from build123d import *

# Parameters (mm, degrees)
F0_W       = 225.552
F0_H       = 9.652
F1_DEPTH   = 19.05
F3_D       = 19.05
F5_W       = 6.35
F5_H       = 260.096
F6_DEPTH   = 19.05
F9_D       = 16.002
F10_W      = 50.8
F10_H      = 25.4
F11_DEPTH  = 22.352
F12_SIZE   = 6.35
F14_D      = 7.9375
F16_D      = 10.3124
F16_DEPTH  = 28.8925
F16_TIP    = 3.0981575238
F18_D      = 10.3124
F18_DEPTH  = 12.7
F18_TIP    = 3.0981575238
F20_DEPTH  = 6.35
F22_SIZE   = 14.224
F22_2_SIZE = 14.224
F23_W      = 38.1
F23_H      = 276.225
F24_DEPTH  = 7.874


with BuildPart() as f1:
    # F0 (on Right) → F1 (new body, symmetric)
    with BuildSketch(Plane.YZ):
        with Locations((0, 134.874)):
            Rectangle(F0_W, F0_H)
    extrude(amount=F1_DEPTH, both=True)

    # F3 (through all)
    with Locations(Plane.XY.offset(139.7)):
        with Locations((0, -96.8375), (0, 96.8375)):
            Hole(F3_D / 2)


with BuildPart() as f4_1:
    # F4: instance of F1
    add(f1.part.mirror(Plane.XY))


with BuildPart() as f6:
    # F5 (on Right) → F6 (new body, symmetric)
    with BuildSketch(Plane.YZ):
        with Locations((-80.9625, 0)):
            Rectangle(F5_W, F5_H)
    extrude(amount=F6_DEPTH, both=True)


with BuildPart() as f6b:
    # F5 (on Right) → F6, piece 2 (new body, symmetric)
    with BuildSketch(Plane.YZ):
        with Locations((80.9625, 0)):
            Rectangle(F5_W, F5_H)
    extrude(amount=F6_DEPTH, both=True)


with BuildPart() as f1_1:
    add(f1.part)

    # F8: union F6, F6b, F4_1
    add(f6.part)
    add(f6b.part)
    add(f4_1.part)

    # F9 (through all)
    with Locations(Plane(origin=(0, 84.1375, 0), x_dir=(-1, 0, 0), z_dir=(0, 1, 0))):
        with Locations((0, -3.048)):
            Hole(F9_D / 2)

    # F10 (on face) → F11 (join)
    with BuildSketch(Plane.XY.offset(-130.048)):
        with Locations((0, -51.689)):
            Rectangle(F10_W, F10_H)
        Rectangle(F10_W, F10_H)
        with Locations((0, 51.689)):
            Rectangle(F10_W, F10_H)
    extrude(amount=F11_DEPTH)

    # F12
    f12_edges = [f1_1.edges().sort_by_distance(p)[0] for p in [
        (-25.4, -51.689, -107.696),
        (-25.4, 0, -107.696),
        (-25.4, 51.689, -107.696),
        (25.4, 51.689, -107.696),
        (25.4, 0, -107.696),
        (25.4, -51.689, -107.696),
    ]]
    chamfer(f12_edges, length=F12_SIZE)

    # F14 (through all)
    with Locations(Plane.XY.offset(139.7)):
        with Locations((0, -34.925), (0, 34.925)):
            Hole(F14_D / 2)

    # F16
    with Locations(Plane.XY.offset(139.7)):
        with Locations((0, 0)):
            Hole(F16_D / 2, depth=F16_DEPTH)
            with Locations((0, 0, -(F16_DEPTH + F16_TIP / 2))):  # 118° drill point
                Cone(0, F16_D / 2, F16_TIP, mode=Mode.SUBTRACT)

    # F18
    with Locations(Plane(origin=(0, 0, -139.7), x_dir=(1, 0, 0), z_dir=(0, 0, -1))):
        with Locations((0, 0)):
            Hole(F18_D / 2, depth=F18_DEPTH)
            with Locations((0, 0, -(F18_DEPTH + F18_TIP / 2))):  # 118° drill point
                Cone(0, F18_D / 2, F18_TIP, mode=Mode.SUBTRACT)

    # F21: F20 across plane


with BuildPart() as f20:
    # F19 (on face) → F20 (new body)
    with BuildSketch(Plane.XY.offset(139.7)):
        Polygon((19.05, 104.902), (19.05, 79.502), (73.2887461782, 79.502), (95.25, 79.502), (95.25, 104.902), align=None)
    extrude(amount=-F20_DEPTH)


with BuildPart() as f1_2:
    add(f1_1.part)
    add(f20.part.mirror(Plane.XY))

    # F22#2
    f22_2_edges = [f1_2.edges().sort_by_distance(p)[0] for p in [
        (95.25, 79.502, -136.525),
    ]]
    chamfer(f22_2_edges, length=F22_2_SIZE)



with BuildPart() as f20_1:
    add(f20.part)

    # F22
    f22_edges = [f20_1.edges().sort_by_distance(p)[0] for p in [
        (95.25, 79.502, 136.525),
    ]]
    chamfer(f22_edges, length=F22_SIZE)


with BuildPart() as f1_3:
    add(f1_2.part)

    add(f20_1.part)  # F24 merges F20
    # F23 (on face) → F24 (join)
    with BuildSketch(Plane(origin=(0, 104.902, 0), x_dir=(-1, 0, 0), z_dir=(0, 1, 0))):
        with Locations((-76.2, -1.5875)):
            Rectangle(F23_W, F23_H)
    extrude(amount=F24_DEPTH)


solid = f1_3.part
Read the model definition and answer for the solid it produces. Units are mm, in the model's axes. A direction names the side the tool comes from. Round coordinates to 2 decimals unless told otherwise and drop trailing zeros. Write each loop counter-clockwise with the first axis right and the second up, starting at its lowest first coordinate (ties: lowest second). Pieces come first, ordered by that corner, then holes. Notation, with made-up numbers: M 4,-15.5 L 56,-15.5 A15 cw 56,6.5 Z; hole C -15,-26.75 d4. An arc over 180 degrees is marked long. Use a Markdown table: item, result.
1) The part is cut by section B-B (z = -97.5). Write down the section's boundary in (x, y), plus the area to 3 significant figures.
Answers follow:
| item | result |
|---|---|
| outline | M -19.05,-84.14 L 19.05,-84.14 L 19.05,-77.79 L -19.05,-77.79 Z; M -19.05,77.79 L 19.05,77.79 L 19.05,84.14 L -19.05,84.14 Z; M 57.15,104.9 L 95.25,104.9 L 95.25,112.78 L 57.15,112.78 Z |
| area | 784 mm2 |
2) The part is cut by section D-D (x = 34). Write down the section's boundary in (y, z).
Answers follow:
| item | result |
|---|---|
| outline | M 79.5,-139.7 L 104.9,-139.7 L 104.9,-133.35 L 79.5,-133.35 Z; M 79.5,133.35 L 104.9,133.35 L 104.9,139.7 L 79.5,139.7 Z |
3) The part is cut by section A-A (y = 42.5). Write down the section's boundary in (x, z), plus the area to 3 significant figures.
Answers follow:
| item | result |
|---|---|
| outline | M -25.4,-130.05 L -19.05,-130.05 L -19.05,-139.7 L 19.05,-139.7 L 19.05,-130.05 L 25.4,-130.05 L 25.4,-114.05 L 19.05,-107.7 L -19.05,-107.7 L -25.4,-114.05 Z; M -19.05,130.05 L 19.05,130.05 L 19.05,139.7 L -19.05,139.7 Z |
| area | 1,830 mm2 |
4) For a pull along Y with two mould halves and no side action, classify faces 5 (the flat face through (0, -112.776, 135)), 6 (the flat face through (0, 26, -130.048)), 7 (the flat face through (0, 112.776, 135)), 8 (the flat face through (9, 101, 130.048)) as pulls with the +Y half, pulls with the -Y half, needs draft (parallel to the pull), parting line crosses it, or undercut.
Answers follow:
| item | result |
|---|---|
| face 5 | pulls with the -Y half |
| face 6 | undercut |
| face 7 | pulls with the +Y half |
| face 8 | needs draft |
5) A tool of negligible diameter and unlimited length cuts with its end or side. For faces 1 (the flat face through (50, 79.502, -137)), 2 (the flat face through (0, 52, -107.696)), 3 (the flat face through (76, 109, 136.525)), 4 (the flat face through (9, -102, 130.048)), from which of +Z, -Z, +X, -X, +Y, -Y can it reach the whole face along a straight path? Write none if from no direction.
Answers follow:
| item | result |
|---|---|
| face 1 | +Z, -Z, +X, -Y |
| face 2 | +X, -X |
| face 3 | +Z, +X, +Y |
| face 4 | +X, -X, -Y |
6) The part is cut by section C-C (x = 14). Write down the section's boundary in (y, z), plus the area to 3 significant figures.
Answers follow:
| item | result |
|---|---|
| outline | M -112.78,-139.7 L 112.78,-139.7 L 112.78,-130.05 L 84.14,-130.05 L 84.14,130.05 L 112.78,130.05 L 112.78,139.7 L -112.78,139.7 L -112.78,130.05 L -84.14,130.05 L -84.14,-130.05 L -112.78,-130.05 Z; hole M -77.79,-130.05 L -64.39,-130.05 L -64.39,-107.7 L -38.99,-107.7 L -38.99,-130.05 L -12.7,-130.05 L -12.7,-107.7 L 12.7,-107.7 L 12.7,-130.05 L 38.99,-130.05 L 38.99,-107.7 L 64.39,-107.7 L 64.39,-130.05 L 77.79,-130.05 L 77.79,130.05 L -77.79,130.05 Z |
| area | 9,360 mm2 |
7) Flat-ended cylindrical pins translate along their axes: pin 1 (13 mm diameter, centred on x = 0, z = -3.048, fed in from +Y); pin 2 (7 mm diameter, centred on x = 24, y = -54.5, fed in from -Z); pin 3 (17.5 mm diameter, centred on y = -54, z = -120.5, fed in from +X); pin 4 (5 mm diameter, centred on x = 61.5, z = 5, fed in from -Y). Find the tip coordinate at first contact, or state that the pin passes through.
Answers follow:
| item | result |
|---|---|
| pin 1 | passes through |
| pin 2 | stops at z = -130.05 |
| pin 3 | stops at x = 25.4 |
| pin 4 | stops at y = 104.9 |
8) Straight lines are drawn through the part: line 1 along Y through (x, z) = (0, 134); line 2 along Z through (x, y) = (12, 53); line 3 along Z through (x, y) = (0, 79). For each, find the intervals that lie inside material, in ascending order. Write a range as [from, to].
Answers follow:
| item | result |
|---|---|
| line 1 | y = [-112.78, -106.36], [-87.31, -38.89], [-30.96, -5.16], [5.16, 30.96], [38.89, 87.31], [106.36, 112.78] |
| line 2 | z = [-139.7, -107.7], [130.05, 139.7] |
| line 3 | z = [-139.7, -11.05], [4.95, 139.7] |
